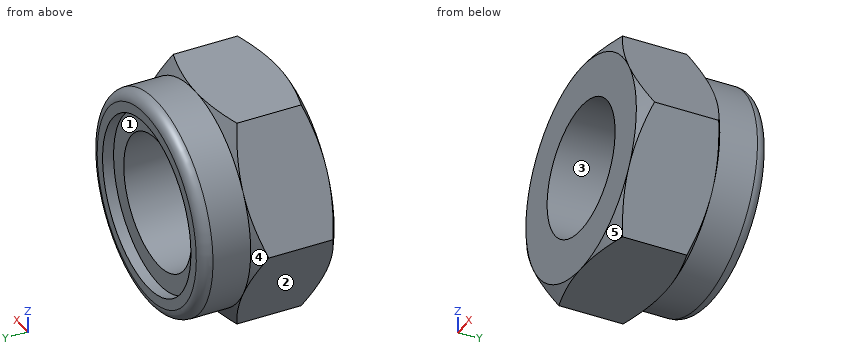
from build123d import *

# Parameters (mm, degrees)
EXTRUDE1_DEPTH     = 2.525
CUT_EXTRUDE1_REACH = 14.751
SKETCH4_R          = 4


with BuildPart() as part:
    # Sketch1 → Extrude1 (new, symmetric)
    with BuildSketch(Plane(origin=(0, 0, 0), x_dir=(1, 0, 0), z_dir=(0, 1, 0))):
        Polygon((3.75277675, 6.5), (-3.75277675, 6.5), (-7.505553499, 0), (-3.75277675, -6.5), (3.75277675, -6.5), (7.505553499, 0), align=None)
    extrude(amount=EXTRUDE1_DEPTH, both=True)

    # Sketch2 → Cut-Revolve1 (revolve, cut)
    with BuildSketch(Plane.XY):
        Polygon((7.505553499, 2.525), (6.5, 2.525), (7.505553499, 1.944443416), align=None)
    cut_revolve1 = revolve(axis=Axis((0, 2.75, 0), (0, -1, 0)), mode=Mode.SUBTRACT)

    # Mirror1: Cut-Revolve1 across plane
    add(cut_revolve1.mirror(Plane.ZX), mode=Mode.SUBTRACT)

    # Sketch3 → Revolve1 (revolve)
    with BuildSketch(Plane.XY, mode=Mode.PRIVATE) as revolve1_sk:
        with BuildLine():
            Line((0, 2.525), (0, 4.808333333))
            Line((0, 4.808333333), (5.2, 4.808333333))
            Line((5.2, 4.808333333), (5.2, 5.475))
            Line((5.2, 5.475), (5.833333333, 5.475))
            ThreePointArc((5.833333333, 5.475), (6.304737854, 5.279737854), (6.5, 4.808333333))
            Line((6.5, 4.808333333), (6.5, 2.525))
            Line((6.5, 2.525), (0, 2.525))
        make_face()
    revolve(revolve1_sk.sketch.rotate(Axis((0, 2.75, 0), (0, -1, 0)), 90), axis=Axis((0, 2.75, 0), (0, -1, 0)))

    # Sketch4 → Cut-Extrude1 (cut, up to next)
    with BuildSketch(Plane.XZ.offset(2.525), mode=Mode.PRIVATE) as cut_extrude1_sk1:
        with Locations(Location((0, 0, 0), (0, 0, 270))):
            Circle(SKETCH4_R)
    cut_extrude1_tool1 = extrude(cut_extrude1_sk1.sketch, amount=-CUT_EXTRUDE1_REACH, mode=Mode.PRIVATE) & part.part
    add(cut_extrude1_tool1.solids().sort_by_distance((0, -2.525, 0))[0], mode=Mode.SUBTRACT)


solid = part.part
Input: part model. Units: mm. Frame: model coordinates. Face numbers are marked on the shaded views. A direction names the side the tool comes from. Coordinates: 2 decimals unless noted, no trailing zeros. Write each loop counter-clockwise with the first axis right and the second up, starting at its lowest first coordinate (ties: lowest second). Pieces come first, ordered by that corner, then holes. Notation, with made-up numbers: M 0,36.25 L 50,36.25 A30 cw 50,71.25 Z; hole C 81,6 d7. An arc over 180 degrees is marked long. Answer as a JSON object with one key per item and string values. Group by question number.
(1) Section A-A on y = -0.25. Output: boundary loops of the cut face in (x, z), plus the area to 3 significant figures.
(2) Ray query, line 1 along Z through (x, y) = (0.25, 0.5); line 2 along X through (y, z) = (-0.5, -2); line 3 along Z through (x, y) = (1.25, 4). Return the intervals inside material, ascending. Write a range as [from, to].
(3) Set-up query: the marked faces 1 and 2. Return all of +Z, -Z, +X, -X, +Y, -Y with unobstructed straight access to the full face (end or side cutting, diameter ignored); none if empty.
(4) Contact query for flat-ended pins moving along their axis: P1, Ø2, axis at y = 1, z = -4, coming from the -X side; P2, Ø2, axis at x = 1.5, y = 3.5, coming from the -Z side; P3, Ø3, axis at y = 0.5, z = -2.5, coming from the -X side. Output: stop coordinate, or through.
(5) Mould query, pull axis Z, two halves, no side actions, for the marked faces 3, 4 and 5. Classes: pulls with the +Z half, pulls with the -Z half, needs draft (parallel to the pull), parting line crosses it, or undercut.
Result set:
{
 "1": {"outline": "M -7.51,0 L -3.75,-6.5 L 3.75,-6.5 L 7.51,0 L 3.75,6.5 L -3.75,6.5 Z; hole C 0,0 d8", "area": "96.1 mm2"},
 "2": {"line 1": "z = [-6.5, -3.99], [3.99, 6.5]", "line 2": "x = [-6.35, -3.46], [3.46, 6.35]", "line 3": "z = [-6.38, -3.8], [3.8, 6.38]"},
 "3": {"face 1": "+Y", "face 2": "-Z, -X, +Y, -Y"},
 "4": {"P1": "stops at x = -5.77", "P2": "stops at z = -6.48", "P3": "stops at x = -6.93"},
 "5": {"face 3": "undercut", "face 4": "parting line crosses it", "face 5": "pulls with the -Z half"}
}
